Can you work these out from the drawing? Everything is in mm from the part's minimum corner. A direction names the side the tool comes from. Coordinates: 2 decimals unless noted, no trailing zeros. Order: outer loops, then holes, each group sorted by start corner. A loop starts at its lowest first (then second) coordinate and runs counter-clockwise, first axis right, second up. Notation, with made-up numbers: M 56.25,-14.5 L 86.25,-14.5 A14 cw 86.25,2.5 Z; hole C 40,5.25 d5. An arc over 180 degrees is marked long. Answer as a JSON object with one key per item and string values.
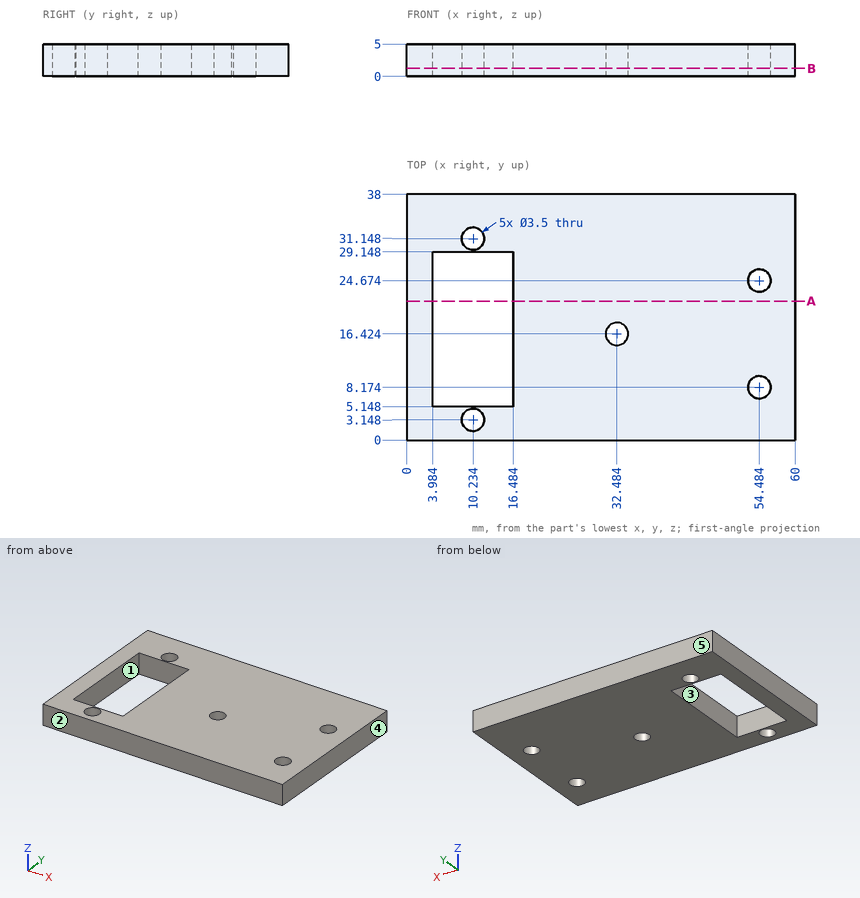
Item 1: Which directions (+Z, -Z, +X, -X, +Y, -Y) give clear straight access to the entire face, cutting with the end or side of a thin tool? Please do the marked faces 1 and 2.
Answers follow:
{"face 1": "+Z, -Z", "face 2": "+Z, -Z, +X, -X, -Y"}
Item 2: Please list where these lines run through material, in increasing order: line 1 (Y direction, x = 7.5, z = 3.5); line 2 (Y direction, x = 32.5, z = 0.55); line 3 (X direction, y = 12.5, z = 3.8).
Answers follow:
{"line 1": "y = 0 to 5.15, 29.15 to 38", "line 2": "y = 0 to 14.67, 18.17 to 38", "line 3": "x = 0 to 3.98, 16.48 to 60"}
Item 3: I want a section at B-B, the plane z = 1.25. Write out the boundary of the cut face in (x, y).
Answers follow:
{"outline": "M 0,0 L 60,0 L 60,38 L 0,38 Z; hole M 3.98,5.15 L 16.48,5.15 L 16.48,29.15 L 3.98,29.15 Z; hole C 10.23,3.15 d3.5; hole C 10.23,31.15 d3.5; hole C 32.48,16.42 d3.5; hole C 54.48,8.17 d3.5; hole C 54.48,24.67 d3.5"}
Item 4: I want a section at A-A, the plane y = 21.5. Write out the boundary of the cut face in (x, z).
Answers follow:
{"outline": "M 0,0 L 3.98,0 L 3.98,5 L 0,5 Z; M 16.48,0 L 60,0 L 60,5 L 16.48,5 Z"}
Item 5: If we mould it in two halves opening along X, with no side actions, what happens to the marked faces 3, 4 and 5? For each: pulls with the +X half, pulls with the -X half, needs draft (parallel to the pull), parting line crosses it, or undercut.
Answers follow:
{"face 3": "undercut", "face 4": "pulls with the +X half", "face 5": "needs draft"}
